Autodesk Inventor part; units mm, degrees
ref_plane "YZ Plane" through (0, 0, 0) normal (1, 0, 0) x (0, 1, 0)
ref_plane "XZ Plane" through (0, 0, 0) normal (0, 1, 0) x (-1, 0, 0)
ref_plane "XY Plane" through (0, 0, 0) normal (0, 0, 1) x (1, 0, 0)
sketch "Sketch1" plane through (0, 0, 0) normal (0, 0, 1) x (1, 0, 0)
  line L0 (-22, -30) -> (22, -30)
  line L1 (22, -30) -> (22, 30)
  line L2 (22, 30) -> (-22, 30)
  line L3 (-22, 30) -> (-22, -30)
  line L4 (-22, -30) -> (22, 30) construction
  line L5 (22, -30) -> (-22, 30) construction
  line L6 (-15, -38) -> (15, -38)
  line L7 (15, -38) -> (15, -30)
  line L8 (15, -30) -> (-15, -30)
  line L9 (-15, -30) -> (-15, -38)
  line L10 (-15, -38) -> (15, -30) construction
  line L11 (15, -38) -> (-15, -30) construction
  circle A0 centre (0, 15) radius 1.65
  point P0 (0, 0)
  point P1 (0, -34)
  point P2 (0, -30)
  point P3 (0, 30)
  dimension "d0" = 44
  dimension "d1" = 60
  dimension "d2" = 30
  dimension "d3" = 8
  dimension "d4" = 3.3
  dimension "d5" = 15
sketch "Sketch2" plane through (0, 0, 5) normal (0, 0, 1) x (1, 0, 0)
  line L0 (22, -30) -> (22, 30)
  line L1 (22, -20) -> (25.5, -20)
  line L2 (25.5, -20) -> (25.5, -8)
  line L3 (25.5, -8) -> (22, -8)
  line L4 (22, -8) -> (22, -20)
  line L5 (22, -30) -> (15, -30)
  line L6 (0, 0) -> (0, -38)
  line L7 (-15, -38) -> (15, -38)
  line L8 (-22, -20) -> (-25.5, -20)
  line L9 (-25.5, -20) -> (-25.5, -8)
  line L10 (-25.5, -8) -> (-22, -8)
  line L11 (-22, -8) -> (-22, -20)
  dimension "d7" = 3.5
  dimension "d8" = 12
  dimension "d9" = 10
extrude "Plate1" add sketch "Sketch1" along normal blind 5
sheet face with bend "Face2" sketch "Sketch2" thickness 5 toward (0, 0, -1) bend radius 5
bend "Bend1"
equation "\"d6\" = Thickness"
equation "\"d10\" = BendRadius"
equation "\"d11\" = BendReliefWidth"
equation "\"d13\" = MinimumRemnant"
equation "\"d12\" = BendReliefDepth"
equation "\"d14\" = TransitionRadius"
equation "\"BendRadius\" = Thickness"
equation "\"BendReliefWidth\" = Thickness"
equation "\"BendReliefDepth\" = 0.5 * Thickness"
equation "\"TransitionRadius\" = BendRadius"
equation "\"JacobiRadiusSize\" = BendRadius"
equation "\"GapSize\" = Thickness"
properties part number "Path Back End"
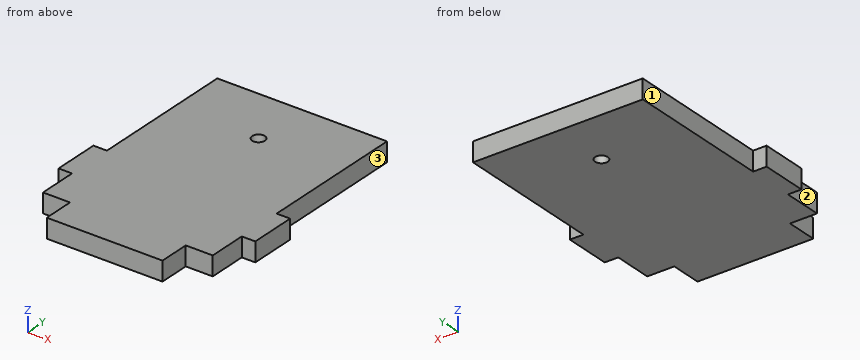
Verification items for the finished model (mm, model axes). Face numbers are marked on the shaded views. A direction names the side the tool comes from. Coordinates: 2 decimals unless noted, no trailing zeros. Write each loop counter-clockwise with the first axis right and the second up, starting at its lowest first coordinate (ties: lowest second). Pieces come first, ordered by that corner, then holes. Notation, with made-up numbers: (83, -4) - (101, -4) arc R19 cw to (101, 30) - close; hole circle Ø2 at (-38.5, 19). An arc over 180 degrees is marked (long way). Write item = value, one per line.
Q1. Cross-section at A-A (y = 15). Enter the section's corners in (x, z), plus the area to 4 significant figures.
Answer:
outline = (-22, 0) - (-1.65, 0) - (-1.65, 5) - (-22, 5) - close; (1.65, 0) - (22, 0) - (22, 5) - (1.65, 5) - close
area = 203.5 mm²
Q2. Material ranges on L1, parallel to Y at x = 0, z = 2.9; L2, parallel to X at y = 23, z = 4.1; L3, parallel to Y at x = 19, z = 0.8, recorded low to high. Write a range as from..to.
Answer:
L1 = -38..13.35, 16.65..30
L2 = -22..22
L3 = -30..30
Q3. Go/stop test with flat-tipped pins: pin 1 Ø1.8 at (x, z) = (24, 3) entering from -Y; pin 2 Ø5.5 at (x, y) = (0, 15) entering from -Z; pin 3 Ø2.5 at (y, z) = (-32, 3.5) entering from -X; pin 4 Ø1 at (y, z) = (-28, 3.5) entering from +X. Record where each tip stops, or that it passes through.
Answer:
pin_1 = -20
pin_2 = 0
pin_3 = -15
pin_4 = 22
Q4. Cross-section at C-C (z = 2.2). Enter the section's corners in (x, y).
Answer:
outline = (-25.5, -20) - (-22, -20) - (-22, -30) - (-15, -30) - (-15, -38) - (15, -38) - (15, -30) - (22, -30) - (22, -20) - (25.5, -20) - (25.5, -8) - (22, -8) - (22, 30) - (-22, 30) - (-22, -8) - (-25.5, -8) - close; hole circle Ø3.3 at (0, 15)
Q5. Cross-section at B-B (x = 0). Enter the section's corners in (y, z), plus the area to 4 significant figures.
Answer:
outline = (-38, 0) - (13.35, 0) - (13.35, 5) - (-38, 5) - close; (16.65, 0) - (30, 0) - (30, 5) - (16.65, 5) - close
area = 323.5 mm²
Q6. Access from +Z, -Z, +X, -X, +Y, -Y to the whole of each face (thin tool, end or side, straight path). Record for the marked faces 1, 2 and 3.
Answer:
face_1 = +Z, -Z, -X, +Y
face_2 = +Z, -Z, -X, -Y
face_3 = +Z, -Z, +X, +Y
Q7. Cross-section at D-D (y = 2). Enter the section's corners in (x, z).
Answer:
outline = (-22, 0) - (22, 0) - (22, 5) - (-22, 5) - close
